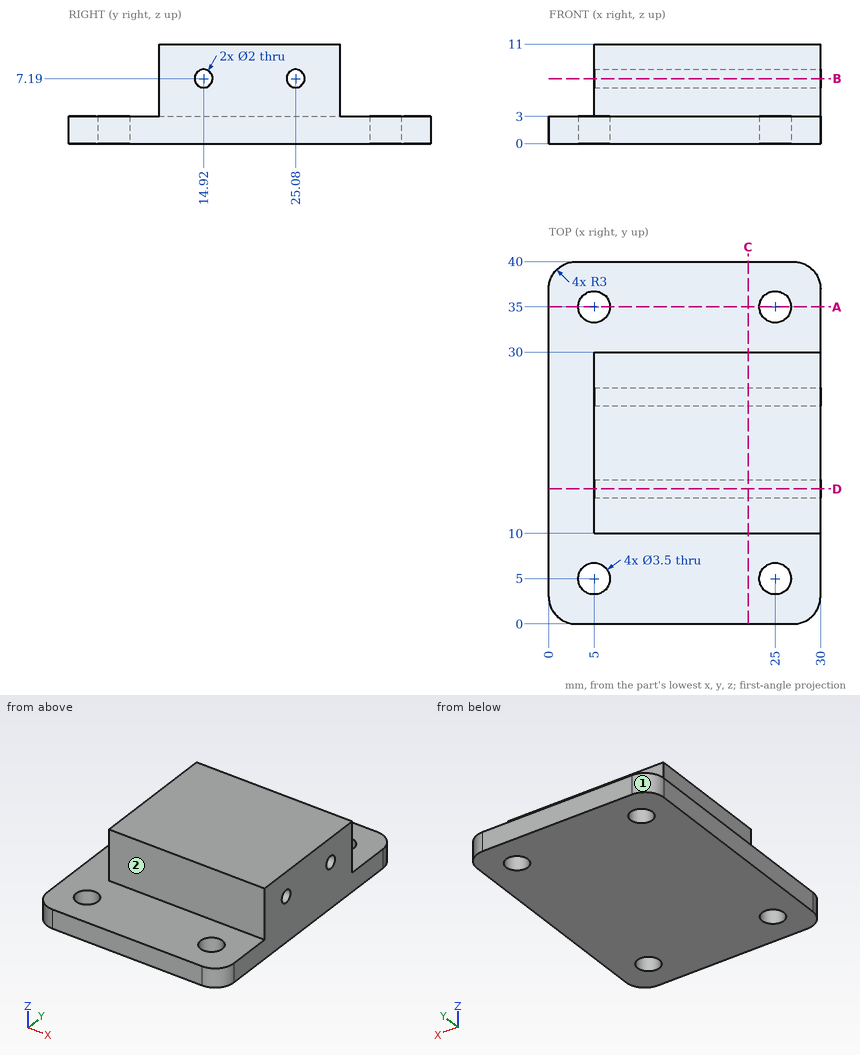
Verification items for this drawing (mm, ordinates from the low corner). A direction names the side the tool comes from. Coordinates: 2 decimals unless noted, no trailing zeros. Loops run counter-clockwise (first coordinate to the right, second up) from the corner with the lowest first, then second, coordinate; pieces in that order, holes last. Notation, with made-up numbers: (76, 13) -> (115, 13) arc R7 ccw to (115, 25) -> close; hole circle Ø1 at (24, 74). An arc over 180 degrees is marked (long way). Put each result on its own line as item: value.
1. Section check C-C, the plane x = 22. Record the boundary of the cut face in (y, z), then the cut area to 3 significant figures.
Result set:
outline: (0, 0) -> (40, 0) -> (40, 3) -> (30, 3) -> (30, 11) -> (10, 11) -> (10, 3) -> (0, 3) -> close; hole circle Ø2 at (14.92, 7.19); hole circle Ø2 at (25.08, 7.19)
area: 274 mm^2
2. Section check D-D, the plane y = 14.92. Record the boundary of the cut face in (x, z), then the cut area to 3 significant figures.
Result set:
outline: (0, 0) -> (30, 0) -> (30, 6.19) -> (5, 6.19) -> (5, 3) -> (0, 3) -> close; (5, 8.19) -> (30, 8.19) -> (30, 11) -> (5, 11) -> close
area: 240 mm^2
3. Gauge pin test, flat ends, axial feed: P1, Ø4, axis at x = 26, y = 6.5, coming from the +Z side; P2, Ø2.5, axis at x = 16, z = 6, coming from the +Y side; P3, Ø4, axis at x = 14, z = 9.5, coming from the -Y side; P4, Ø3, axis at x = 25, y = 5, coming from the +Z side. Record the tip position at first contact, or that the pin passes through.
Result set:
P1: stops at z = 3
P2: stops at y = 30
P3: stops at y = 10
P4: passes through
4. Section check A-A, the plane y = 35. Record the boundary of the cut face in (x, z), then the cut area to 3 significant figures.
Result set:
outline: (0, 0) -> (3.25, 0) -> (3.25, 3) -> (0, 3) -> close; (6.75, 0) -> (23.25, 0) -> (23.25, 3) -> (6.75, 3) -> close; (26.75, 0) -> (30, 0) -> (30, 3) -> (26.75, 3) -> close
area: 69.0 mm^2
5. Thickness scan on line 1 (Y direction, x = 5, z = 0.6); line 2 (Y direction, x = 24.75, z = 7.19); line 3 (Y direction, x = 13, z = 10.5). Record the ranges inside material, lowest first.
Result set:
line 1: y = 0 to 3.25, 6.75 to 33.25, 36.75 to 40
line 2: y = 10 to 13.92, 15.92 to 24.08, 26.08 to 30
line 3: y = 10 to 30
6. Section check B-B, the plane z = 7.19. Record the boundary of the cut face in (x, y).
Result set:
outline: (5, 10) -> (30, 10) -> (30, 13.92) -> (5, 13.92) -> close; (5, 15.92) -> (30, 15.92) -> (30, 24.08) -> (5, 24.08) -> close; (5, 26.08) -> (30, 26.08) -> (30, 30) -> (5, 30) -> close
7. Tool access check on the marked faces 1 and 2. Record the directions out of +Z, -Z, +X, -X, +Y, -Y that give a thin tool (end or side, any length) a straight path to the whole face; none if there is none.
Result set:
face 1: +Z, -Z, -X, +Y
face 2: +Z, +X, -X, -Y
